Here's how the part is built. I have some questions about the finished solid (model axes, mm). Face numbers are marked on the shaded views. A direction names the side the tool comes from. Round coordinates to 2 decimals unless told otherwise and drop trailing zeros. Write each loop counter-clockwise with the first axis right and the second up, starting at its lowest first coordinate (ties: lowest second). Pieces come first, ordered by that corner, then holes. Notation, with made-up numbers: (2.5, -17) - (45.5, -17) arc R15 cw to (45.5, -12) - close; hole circle Ø4 at (38, 80). An arc over 180 degrees is marked (long way). One line per question, with ' | ' between items. Start each with the question number.
(1) Imagine slicing it at A-A (x = 30). Write out the boundary of the cut face in (y, z).
(2) For the marked faces 1 and 2, which set-ups out of +Z, -Z, +X, -X, +Y, -Y let a thin tool reach every point of the face, with its end or its side?
(3) If I drill on L1, parallel to Z at x = 28, y = -34; L2, parallel to Y at x = 29.5, z = -12; L3, parallel to X at y = -24, z = -2.5, over which ranges is the centre line in solid material (lowest first)?
(4) Imagine slicing it at D-D (x = 20.5). Write out the boundary of the cut face in (y, z).
(5) Will these pins go through, and if not, where does the flat tip stop? pin 1 (1.5 mm diameter, centred on x = 29.5, z = -1.5, fed in from +Y); pin 2 (5 mm diameter, centred on x = 11.5, y = -31, fed in from +Z); pin 3 (6 mm diameter, centred on y = -19, z = 6, fed in from +X); pin 4 (2 mm diameter, centred on y = -29.5, z = -21, fed in from +X).
(6) Imagine slicing it at C-C (z = 3). Write out the boundary of the cut face in (x, y), plus the area to 3 significant figures.
(7) Imagine slicing it at B-B (z = -21). Write out the boundary of the cut face in (x, y).
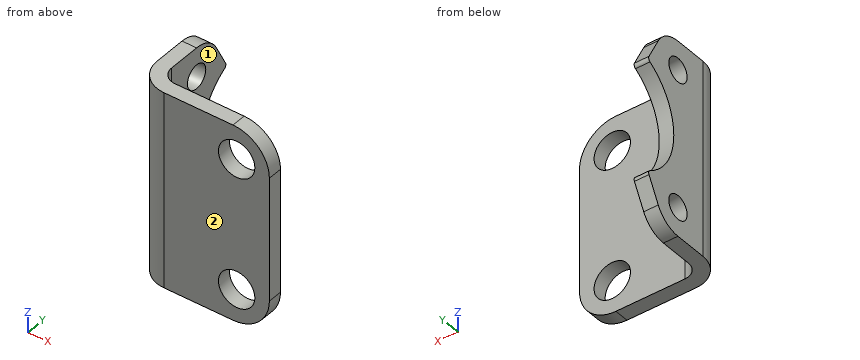
Autodesk Inventor part; units mm, degrees
ref_plane "HNC_1_XY" through (0, 0, 0) normal (1, 0, 0) x (0, 0, -1)
ref_plane "HNC_1_YZ" through (0, 0, 0) normal (0, 0, -1) x (0, 1, 0)
ref_plane "HNC_1_ZX" through (0, 0, 0) normal (0, 1, 0) x (1, 0, 0)
sketch "Sketch_1" plane through (0, 0, 0) normal (0, 0, 1) x (1, 0, 0)
  line L0 (0, -1) -> (0, -28)
  arc A0 (0, -28) -> (8, -36) centre (8, -28) ccw
  line L1 (8, -36) -> (37, -36)
  line L2 (37, -36) -> (37, -32)
  line L3 (37, -32) -> (8, -32)
  arc A1 (4, -28) -> (8, -32) centre (8, -28) ccw
  line L4 (4, -28) -> (4, -1)
  line L5 (4, -1) -> (0, -1)
extrude "Extrusion1" add sketch "Sketch_1" along normal mid plane 54
sketch "Sketch_2" plane through (0, 0, 0) normal (0, 1, 0) x (-1, 0, 0)
  line L0 (-27, -37) -> (-27, -27)
  arc A0 (-37, -17) -> (-27, -27) centre (-27, -17) ccw
  line L1 (-37, -17) -> (-37, 17)
  arc A1 (-27, 27) -> (-37, 17) centre (-27, 17) ccw
  line L2 (-27, 27) -> (-27, 37)
  line L3 (-27, 37) -> (-47, 37)
  line L4 (-47, 37) -> (-47, -37)
  line L5 (-47, -37) -> (-27, -37)
extrude "Extrusion2" cut sketch "Sketch_2" along normal mid plane 74
sketch "Sketch_3" plane through (0, 0, 0) normal (0, 1, 0) x (-1, 0, 0)
  circle A0 centre (-28, -18) radius 5
extrude "Extrusion3" cut sketch "Sketch_3" along normal mid plane 74
sketch "Sketch_4" plane through (0, 0, 0) normal (0, 1, 0) x (-1, 0, 0)
  circle A0 centre (-28, 18) radius 5
extrude "Extrusion4" cut sketch "Sketch_4" along normal mid plane 74
sketch "Sketch_5" plane through (0, 0, 0) normal (1, 0, 0) x (0, 1, 0)
  circle A0 centre (-19, 19) radius 3.3
extrude "Extrusion5" cut sketch "Sketch_5" along normal mid plane 10
sketch "Sketch_6" plane through (0, 0, 0) normal (1, 0, 0) x (0, 1, 0)
  circle A0 centre (-19, -19) radius 3.3
extrude "Extrusion6" cut sketch "Sketch_6" along normal mid plane 10
sketch "Sketch_7" plane through (0, 0, 0) normal (1, 0, 0) x (0, 1, 0)
  line L0 (-41, 32) -> (-41, -32)
  line L1 (-41, -32) -> (0, -32)
  line L2 (0, -32) -> (0, 32)
  line L3 (0, 32) -> (-41, 32)
  line L4 (-19, 27) -> (-36, 27)
  line L5 (-36, 27) -> (-36, -27)
  line L6 (-36, -27) -> (-19, -27)
  arc A0 (-19, -27) -> (-11.9155, -22.7161) centre (-19, -19) ccw
  line L7 (-11.9155, -22.7161) -> (-8.5809, -16.359)
  arc A1 (-8.5809, -16.359) -> (-8.9548, -15.0353) centre (-9.4665, -15.8945) ccw
  arc A2 (-8.9548, 15.0353) -> (-8.9548, -15.0353) centre (0, 0) ccw
  arc A3 (-8.9548, 15.0353) -> (-8.5809, 16.359) centre (-9.4665, 15.8945) ccw
  line L8 (-8.5809, 16.359) -> (-11.9155, 22.7161)
  arc A4 (-11.9155, 22.7161) -> (-19, 27) centre (-19, 19) ccw
extrude "Extrusion7" cut sketch "Sketch_7" along normal mid plane 10
ref_plane "HNC_1_XY" through (0, 0, 0) normal (1, 0, 0) x (0, 0, -1)
ref_plane "HNC_1_YZ" through (0, 0, 0) normal (0, 0, -1) x (0, 1, 0)
ref_plane "HNC_1_ZX" through (0, 0, 0) normal (0, 1, 0) x (1, 0, 0)
ref_plane "HNC_2_XY" through (4, -19, 19) normal (1, 0, 0) x (0, 0, -1)
ref_plane "HNC_2_YZ" through (4, -19, 19) normal (0, 0, -1) x (0, 1, 0)
ref_plane "HNC_2_ZX" through (4, -19, 19) normal (0, 1, 0) x (1, 0, 0)
ref_plane "HNC_3_XY" through (4, -19, -19) normal (1, 0, 0) x (0, 0, -1)
ref_plane "HNC_3_YZ" through (4, -19, -19) normal (0, 0, -1) x (0, 1, 0)
ref_plane "HNC_3_ZX" through (4, -19, -19) normal (0, 1, 0) x (1, 0, 0)
ref_plane "P19_XY" through (28, -32, -18) normal (0, 1, 0) x (1, 0, 0)
ref_plane "P19_YZ" through (28, -32, -18) normal (1, 0, 0) x (0, 0, -1)
ref_plane "P19_ZX" through (28, -32, -18) normal (0, 0, -1) x (0, 1, 0)
ref_plane "P20_XY" through (28, -32, 18) normal (0, 1, 0) x (1, 0, 0)
ref_plane "P20_YZ" through (28, -32, 18) normal (1, 0, 0) x (0, 0, -1)
ref_plane "P20_ZX" through (28, -32, 18) normal (0, 0, -1) x (0, 1, 0)
properties part number "174370 HNC-40---(F)"
Check sheet entries:
1) outline: (-36, -26.54) - (-32, -26.54) - (-32, -22.58) - (-36, -22.58) - close; (-36, -13.42) - (-32, -13.42) - (-32, 13.42) - (-36, 13.42) - close; (-36, 22.58) - (-32, 22.58) - (-32, 26.54) - (-36, 26.54) - close
2) face 1: +Z, -Z, +X, +Y | face 2: +Z, -Z, +X, -X, -Y
3) L1: -26.95 to -23, -13 to 13, 23 to 26.95 | L2: -36 to -32 | L3: 0 to 4
4) outline: (-36, -27) - (-32, -27) - (-32, 27) - (-36, 27) - close
5) pin 1: y = -32 | pin 2: z = 27 | pin 3: x = 4 | pin 4: x = 4.88
6) outline: (0, -28) arc R8 ccw to (8, -36) - (37, -36) - (37, -32) - (8, -32) arc R4 cw to (4, -28) - (4, -17.24) - (0, -17.24) - close | area: 197 mm^2
7) outline: (0, -28) arc R8 ccw to (8, -36) - (24, -36) - (24, -32) - (8, -32) arc R4 cw to (4, -28) - (4, -21.62) - (0, -21.62) - close; (0, -16.38) - (4, -16.38) - (4, -11.02) - (0, -11.02) - close; (32, -36) - (36.17, -36) - (36.17, -32) - (32, -32) - close
